Autodesk Inventor part; units mm, degrees
ref_plane "YZ Plane" through (0, 0, 0) normal (1, 0, 0) x (0, 1, 0)
ref_plane "XZ Plane" through (0, 0, 0) normal (0, 1, 0) x (-1, 0, 0)
ref_plane "XY Plane" through (0, 0, 0) normal (0, 0, 1) x (1, 0, 0)
sketch "スケッチ1" plane through (0, 0, 0) normal (1, 0, 0) x (0, 1, 0)
  line L0 (0, 0) -> (20.1, 0)
  line L1 (20.1, 0) -> (20.1, -20)
  line L2 (20.1, -20) -> (0, -20)
  line L3 (0, -20) -> (0, 0)
  line L4 (0, -20) -> (5, -20)
  line L5 (5, -20) -> (5, -95)
  line L6 (5, -95) -> (0, -95)
  line L7 (0, -95) -> (0, -20)
  circle A0 centre (2.5, -38) radius 1.5
  circle A1 centre (2.5, -56) radius 1.5
  circle A2 centre (2.5, -74) radius 1.5
  line L8 (20.1, 0) -> (25.1, 0)
  line L9 (25.1, 0) -> (25.1, -20)
  line L10 (25.1, -20) -> (20.1, -20)
  line L11 (20.1, -20) -> (20.1, 0)
  line L12 (0, 0) -> (-5, 0)
  line L13 (-5, 0) -> (-5, -20)
  line L14 (-5, -20) -> (0, -20)
  line L15 (0, -20) -> (0, 0)
  line L16 (25.1, -20) -> (5, -95)
  line L17 (-5, -20) -> (0, -95)
  line L18 (25.1, -25) -> (15.1, -25)
  line L19 (15.1, -25) -> (15.1, 0.1)
  line L20 (0, -25) -> (25.1, -25)
  line L21 (25.1, -25) -> (25.1, 0.1)
  line L22 (20.2704, -18.7057) -> (0.1704, -93.7057)
  line L23 (7, -95) -> (7, -18)
  line L24 (7, -18) -> (0, -18)
  line L25 (0, -35) -> (-35, -35)
  line L26 (-35, -35) -> (-35, -85)
  line L27 (-35, -85) -> (0, -85)
  line L28 (0, -85) -> (0, -35)
  line L29 (-35, -38) -> (-70, -38)
  line L30 (-70, -38) -> (-70, -82)
  line L31 (-70, -82) -> (-35, -82)
  line L32 (-35, -82) -> (-35, -38)
  line L33 (7.5, -95) -> (-2.5, -95)
  line L34 (-2.5, -95) -> (-2.5, -21)
  line L35 (-2.5, -21) -> (7.5, -21)
  line L36 (7.5, -21) -> (7.5, -95)
  line L37 (-2.5, -21) -> (-64, -21)
  line L38 (-64, -21) -> (-64, -31)
  line L39 (-64, -31) -> (-2.5, -31)
  line L40 (-2.5, -31) -> (-2.5, -21)
  point P0 (7, -25)
  point P1 (18.5836, -25)
  point P2 (7, -68.2222)
  dimension "d0" = 20.1
  dimension "d1" = 20
  dimension "d2" = 5
  dimension "d3" = 75
  dimension "d4" = 3
  dimension "d5" = 3
  dimension "d6" = 3
  dimension "d7" = 2.5
  dimension "d8" = 2.5
  dimension "d9" = 2.5
  dimension "d10" = 18
  dimension "d11" = 18
  dimension "d12" = 18
  dimension "d13" = 5
  dimension "d14" = 5
  dimension "d15" = 0
  dimension "d16" = 0
  dimension "d17" = 5
  dimension "d18" = 5
  dimension "d19" = 5
  dimension "d20" = 2
  dimension "d33" = 50
  dimension "d34" = 35
  dimension "d35" = 35
  dimension "d36" = 44
  dimension "d37" = 3
  dimension "d38" = 0
  dimension "d39" = 10
  dimension "d40" = 0
  dimension "d41" = 5
  dimension "d42" = 5
  dimension "d43" = 6
  dimension "d44" = 10
  dimension "d46" = 1
extrude "押し出し1" add sketch "スケッチ1" against normal blind 5 contours L3 L14 L13 L12 | L8 L9 L10 L1 | L19 L20 L36 L35 L23 L2 | L2 L22 L18 L19 | L2 L5 L35 L7 | L7 L35 L37 L17 L14 | L2 L10 L16 L18 L22 | L23 L35 L5 L2 | L35 L5 L20 L7 | L7 L25 L34 L35 | L37 L34 L39 L17 | L18 L16 L36 L22 | L35 L36 L20 L23 | L23 L20 L5 L35 | L20 L5 L6 L7 | L39 L34 L25 L17 | L36 L16 L23 L22 | L23 L22 L5 L20 | L7 L27 L17 L34 L25 | L25 L34 L17 | L23 L16 L5 L22 | L7 L17 L27
fillet "フィレット1" radius 2 9 edges at (-2.5, 7, -25) (-2.5, 18.5836, -25) (-2.5, 7, -68.2222) (-2.5, 25.1, 0) (-2.5, 25.1, -20) (-2.5, -5, 0) (-2.5, -5, -20) (-2.5, 0, -95) (-2.5, 5, -95)
sketch "スケッチ2" plane through (0, 25.1, 0) normal (0, 1, 0) x (1, 0, 0)
  line L0 (0, 0) -> (-5, 0)
  line L1 (-5, 2) -> (-5, 19.7366)
  point P0 (-2.5, 10)
  point P1 (-5, 20.1)
  dimension "d24" = 10
  dimension "d25" = 2.5
hole "穴1" at (-2.5, 25.1, -10) direction (0, -1, 0) diameter 3 end through all
equation "\"d8\" = d7"
equation "\"d9\" = d7"
equation "\"d11\" = d10"
equation "\"d12\" = d10"
properties part number "base_weel-v2-Plate-7" material "アルミニウム 6061"
Check sheet for the modelled part. Datum: model origin and axes. Units: mm. A direction names the side the tool comes from. Round coordinates to 2 decimals unless told otherwise and drop trailing zeros. Order: outer loops, then holes, each group sorted by start corner. A loop starts at its lowest first (then second) coordinate and runs counter-clockwise, first axis right, second up.
1) Tool access check on faces 1 (the flat face through (-2, 22, 0)), 2 (the flat face through (-0.8, 20.1, -9.9)), 3 (the flat face through (-2, 12, -25)). Record the directions out of +Z, -Z, +X, -X, +Y, -Y that give a thin tool (end or side, any length) a straight path to the whole face; none if there is none.
2) Section check C-C (y = 8). Record the boundary of the cut face in (x, z), and give its area (3 significant figures).
3) Section check D-D (z = -38). Record the boundary of the cut face in (x, y), and give its area (3 significant figures).
4) Go/stop test with flat-tipped pins: pin 1 Ø1.8 at (x, z) = (-2.5, -10) entering from -Y; pin 2 Ø2.5 at (x, y) = (-3.5, 12) entering from +Z; pin 3 Ø2 at (x, z) = (-1, -49.5) entering from -Y; pin 4 Ø2 at (x, z) = (-4, -59.5) entering from +Y. Record where each tip stops, or that it passes through.
5) Section check A-A (x = -2.5). Give the number of separate pieces and of enclosed holes in the cut face, and give its area (3 significant figures).
6) Section check B-B (z = -10). Record the boundary of the cut face in (x, y).
7) Mould release check, pull along Y, two halves, no side actions. Record for faces 4 (the flat face through (-2.46, 14.47, -40.35)), 5 (the cylindrical face through (-2.54, -4.43, -0.6)), 6 (the flat face through (-5, 6, -47)), 7 (the flat face through (-1, 25.1, -11)): +Y half, -Y half, draft (parallel to the pull), parting line (faces both ways), or undercut.
8) Scan lines: line 1 (Z direction, x = -3, y = 2.5); line 2 (Y direction, x = -1.7, z = -17.5); line 3 (X direction, y = -2.75, z = -10). Record each from-to range of solid material in increasing order.
Result:
1. face 1: +Z, +X, -X, +Y, -Y
1. face 2: +Z, +X, -X
1. face 3: +X, -X
2. outline: (-5, -83.81) - (0, -83.81) - (0, -54.77) - (-5, -54.77) - close; (-5, -25.27) - (0, -25.27) - (0, -20) - (-5, -20) - close
2. area: 172 mm2
3. outline: (-5, -3.8) - (0, -3.8) - (0, 1) - (-5, 1) - close; (-5, 4) - (0, 4) - (0, 7) - (-5, 7) - close; (-5, 15.1) - (0, 15.1) - (0, 20.28) - (-5, 20.28) - close
3. area: 64.9 mm2
4. pin 1: passes through
4. pin 2: stops at z = -20
4. pin 3: stops at y = -3.1
4. pin 4: stops at y = 14.78
5. separate pieces: 3
5. enclosed holes: 4
5. area: 1,240 mm2
6. outline: (-5, -5) - (-4, -5) - (-4, 0) - (-5, 0) - close; (-5, 20.1) - (-4, 20.1) - (-4, 25.1) - (-5, 25.1) - close; (-1, -5) - (0, -5) - (0, 0) - (-1, 0) - close; (-1, 20.1) - (0, 20.1) - (0, 25.1) - (-1, 25.1) - close
7. face 4: undercut
7. face 5: -Y half
7. face 6: draft
7. face 7: +Y half
8. line 1: z = -95 to -75.5, -72.5 to -57.5, -54.5 to -39.5, -36.5 to -20
8. line 2: y = -5 to 0, 20.1 to 25.1
8. line 3: x = -5 to -4, -1 to 0
